Model file for the job. Use its own axes, mm. Face numbers are marked on the shaded views. Give positions to 0.01 mm unless a question says otherwise; leave off trailing zeros. Order: outer loops, then holes, each group sorted by start corner. A loop starts at its lowest first (then second) coordinate and runs counter-clockwise, first axis right, second up. Notation, with made-up numbers: (-32, -39) -> (-15, -39) arc R17 cw to (-15, -12) -> close; hole circle Ø8 at (14, 20). An arc over 180 degrees is marked (long way). Use CSV: the item, a comma, the result in double quotes. Start each with the question number.
1. Cut at B-B on x = 0. List the corners of the cut face in (y, z).
2. Wall check: line 1 (Y direction, x = 0, z = 12.5); line 2 (X direction, y = -1.5, z = 19); line 3 (X direction, y = 0, z = 3.5). Give the ranges that are in metal, low to high. Write a range as from..to.
3. Cut at A-A on z = 16.75. List the corners of the cut face in (x, y).
4. Pull direction Y, two halves, no side cores. Call the marked faces 1, 2, 3 and 4: released by +Y, released by -Y, zero draft, split by the parting line, or undercut.
5. Drop flat-ended pins along their axis: pin 1 (3 mm diameter, centred on y = 0.5, z = 3.5, fed in from +X); pin 2 (8 mm diameter, centred on y = 2.5, z = 7.5, fed in from +X); pin 3 (6 mm diameter, centred on x = 5.5, y = 10.5, fed in from -Z); pin 4 (2 mm diameter, centred on x = 8.5, z = 18, fed in from +Y). Give the stop position or say it passes through.
Autodesk Fusion 360 part; units mm, degrees
sketch "Sketch1" plane through (0, 0, 0) normal (0, 0, 1) x (1, 0, 0)
  line L0 (9.8058, 12.389) -> (-5.8263, 14.6865)
  line L1 (-5.8263, 14.6865) -> (-15.6321, 2.2975)
  line L2 (-15.6321, 2.2975) -> (-9.8058, -12.389)
  line L3 (-9.8058, -12.389) -> (5.8263, -14.6865)
  line L4 (5.8263, -14.6865) -> (15.6321, -2.2975)
  line L5 (15.6321, -2.2975) -> (9.8058, 12.389)
  circle A0 centre (0, 0) radius 4
  dimension "d2" = 15.8
  dimension "d4" = 8
extrude "Extrude1" add sketch "Sketch1" along normal blind 20
sketch "Sketch2" plane through (12.7189, 5.0457, 0) normal (0.9295, 0.3688, 0) x (-0.3688, 0.9295, 0)
  line L0 (-7.9, 0) -> (7.9, 0)
  line L1 (7.9, 0) -> (7.9, 20)
  line L2 (7.9, 20) -> (-7.9, 20)
  line L3 (-7.9, 20) -> (-7.9, 0)
  circle A0 centre (0, 10) radius 2
  dimension "d10" = 4
  dimension "d11" = 10
  dimension "d12" = 7.9
extrude "Extrude2" cut sketch "Sketch2" against normal blind 115.8 contours A0
equation "hub_nut_polygon_radius = 7.9 mm"
equation "d2 = hub_nut_polygon_radius * 2"
equation "center_hole_radius = 4 mm"
equation "d4 = center_hole_radius * 2"
equation "thickness = 20 mm"
equation "extra = 100 mm"
equation "dowel_pin_hole_radius = 2 mm"
equation "d8 = thickness"
equation "d10 = dowel_pin_hole_radius * 2"
equation "d11 = thickness / 2"
equation "d12 = hub_nut_polygon_radius"
equation "d13 = -( hub_nut_polygon_radius * 2 + extra )"
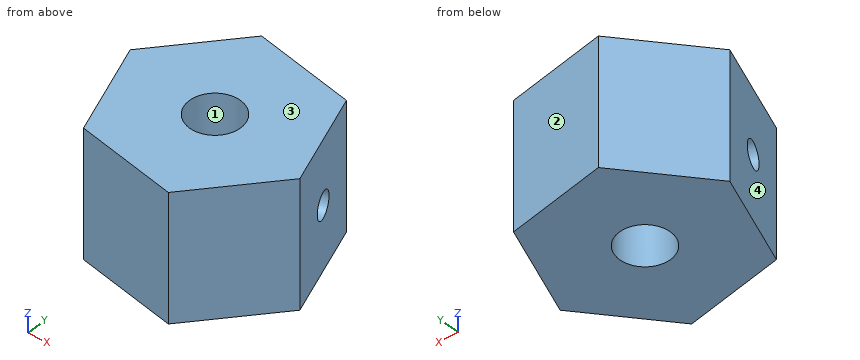
Verdict:
1,outline,"(-13.83, 0) -> (-4, 0) -> (-4, 20) -> (-13.83, 20) -> close; (4, 0) -> (13.83, 0) -> (13.83, 20) -> (4, 20) -> close"
2,line 1,"-13.83..-4, 4..13.83"
2,line 2,"-14.13..-3.71, 3.71..15.32"
2,line 3,"-14.72..-4, 4..14.72"
3,outline,"(-15.63, 2.3) -> (-9.81, -12.39) -> (5.83, -14.69) -> (15.63, -2.3) -> (9.81, 12.39) -> (-5.83, 14.69) -> close; hole circle Ø8 at (0, 0)"
4,face 1,"undercut"
4,face 2,"released by +Y"
4,face 3,"zero draft"
4,face 4,"released by -Y"
5,pin 1,"x = 15.12"
5,pin 2,"x = 15.32"
5,pin 3,"z = 0"
5,pin 4,"y = 12.73"
